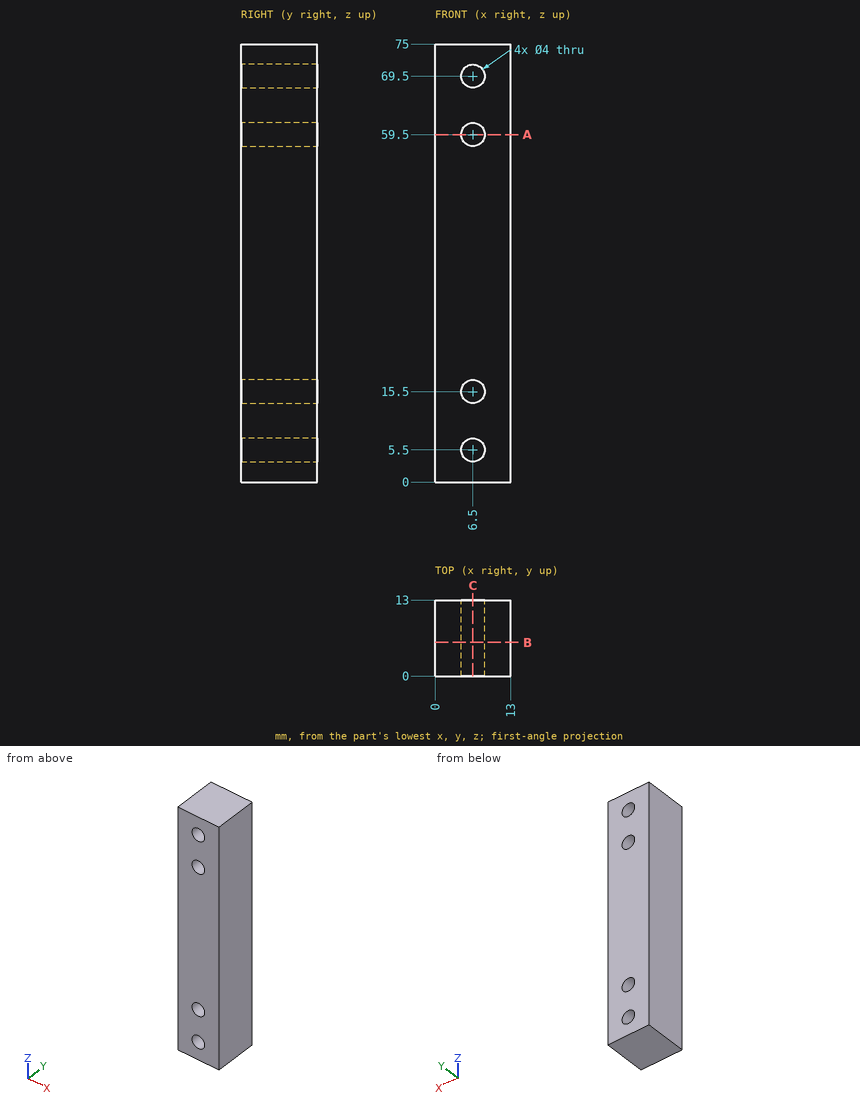
Check sheet for the drawn part. Datum: minimum x, y, z corner. Units: mm. Give positions to 0.01 mm unless a question says otherwise; leave off trailing zeros. Order: outer loops, then holes, each group sorted by start corner. A loop starts at its lowest first (then second) coordinate and runs counter-clockwise, first axis right, second up. Notation, with made-up numbers: (79, -37.5) - (115, -37.5) arc R17 cw to (115, -16.5) - close; hole circle Ø11 at (-21, 2). An arc over 180 degrees is marked (long way). Answer in a Markdown table with one row per item. Add a question column.
Q1. Cross-section at B-B, the plane y = 5.75. Enter the section's corners in (x, z), then the cut area to 3 significant figures.
Q2. Gauge pin test, flat end, axial feed: pin 1 (3.5 mm diameter, centred on x = 6.5, z = 69.5, fed in from -Y). Record the tip position at first contact, or that the pin passes through.
Q3. Material ranges on probe 1 along X at (y, z) = (10.25, 15.5); probe 2 along Z at (x, y) = (7.5, 1); probe 3 along Z at (x, y) = (5, 8), recorded low to high. Write a range as from..to.
Q4. Cross-section at C-C, the plane x = 6.5. Enter the section's corners in (y, z), then the cut area to 3 significant figures.
Q5. Cross-section at A-A, the plane z = 59.5. Enter the section's corners in (x, y), then the cut area to 3 significant figures.
Check values:
| question | item | result |
|---|---|---|
| 1 | outline | (0, 0) - (13, 0) - (13, 75) - (0, 75) - close; hole circle Ø4 at (6.5, 5.5); hole circle Ø4 at (6.5, 15.5); hole circle Ø4 at (6.5, 59.5); hole circle Ø4 at (6.5, 69.5) |
| 1 | area | 925 mm^2 |
| 2 | pin 1 | passes through |
| 3 | probe 1 | x = 0..4.5, 8.5..13 |
| 3 | probe 2 | z = 0..3.77, 7.23..13.77, 17.23..57.77, 61.23..67.77, 71.23..75 |
| 3 | probe 3 | z = 0..4.18, 6.82..14.18, 16.82..58.18, 60.82..68.18, 70.82..75 |
| 4 | outline | (0, 0) - (13, 0) - (13, 3.5) - (0, 3.5) - close; (0, 7.5) - (13, 7.5) - (13, 13.5) - (0, 13.5) - close; (0, 17.5) - (13, 17.5) - (13, 57.5) - (0, 57.5) - close; (0, 61.5) - (13, 61.5) - (13, 67.5) - (0, 67.5) - close; (0, 71.5) - (13, 71.5) - (13, 75) - (0, 75) - close |
| 4 | area | 767 mm^2 |
| 5 | outline | (0, 0) - (4.5, 0) - (4.5, 13) - (0, 13) - close; (8.5, 0) - (13, 0) - (13, 13) - (8.5, 13) - close |
| 5 | area | 117 mm^2 |
